Source: CAD feature listing. Evaluate the final solid. Frame: model axes, mm. A direction names the side the tool comes from. Round coordinates to 2 decimals unless told otherwise and drop trailing zeros. Loops run counter-clockwise (first coordinate to the right, second up) from the corner with the lowest first, then second, coordinate; pieces in that order, holes last. Notation, with made-up numbers: (-28, 53.25) - (-10, 53.25) arc R10 ccw to (-10, 72.25) - close; hole circle Ø7 at (-39.75, 32.5). An arc over 180 degrees is marked (long way). One line per question, with ' | ' between items.
from build123d import *

# Parameters (mm, degrees)
F0_R     = 2.65
F0_R_2   = 3.5
F1_DEPTH = 9.5
F2_DEPTH = 6.35
F3_DEPTH = 9.501


with BuildPart() as f1:
    # F0 (on Top) → F1 (new body)
    with BuildSketch(Plane.XY):
        with Locations((4.775, -2.49704)):
            Circle(F0_R)
        with Locations((5, -2.886751)):
            Circle(F0_R_2)
        with Locations((4.775, -2.49704)):
            Circle(F0_R, mode=Mode.SUBTRACT)
    extrude(amount=F1_DEPTH)

    # F0 (on Top) → F2 (join)
    with BuildSketch(Plane.XY):
        Polygon((1.633975, 0.943376), (0, 0), (0, -5.773503), (5, -8.660254), (10, -5.773503), (10, 0), (5, 2.886751), (3.366025, 1.943376), (3, 0.57735), align=None)
        with Locations((5, -2.886751)):
            Circle(F0_R_2, mode=Mode.SUBTRACT)
    extrude(amount=F2_DEPTH)

    # F0 (on Top) → F3 (cut, through all)
    with BuildSketch(Plane.XY):
        with Locations((4.775, -2.49704)):
            Circle(F0_R)
    extrude(amount=F3_DEPTH, mode=Mode.SUBTRACT)


solid = f1.part
1. Section query A-A, the plane x = 2.75. Return loops of the section in (y, z).
Worked out:
outline: (-7.36, 0) - (-4.21, 0) - (-4.21, 9.5) - (-5.57, 9.5) - (-5.57, 6.35) - (-7.36, 6.35) - close; (-0.79, 0) - (0.64, 0) - (0.64, 6.35) - (-0.21, 6.35) - (-0.21, 9.5) - (-0.79, 9.5) - close
2. Contact query for flat-ended pins moving along their axis: P1, Ø1, axis at x = 3, z = 2.5, coming from the -Y side; P2, Ø5, axis at x = 4.78, y = -2.5, coming from the +Z side; P3, Ø1.5, axis at y = -2.5, z = 8.5, coming from the +X side. Output: stop coordinate, or through.
Worked out:
P1: stops at y = -7.79 | P2: passes through | P3: stops at x = 8.5
3. Material intervals for probe 1 along Z at (x, y) = (7, -6.75); probe 2 along X at (y, z) = (-3, 4.5); probe 3 along X at (y, z) = (-3.75, 2.25), sorted ascending.
Worked out:
probe 1: z = 0 to 6.35 | probe 2: x = 0 to 2.17, 7.38 to 10 | probe 3: x = 0 to 2.44, 7.11 to 10
4. Section query D-D, the plane x = 8. Return loops of the section in (y, z), plus the area to 3 significant figures.
Worked out:
outline: (-6.93, 0) - (1.15, 0) - (1.15, 6.35) - (-1.08, 6.35) - (-1.08, 9.5) - (-4.69, 9.5) - (-4.69, 6.35) - (-6.93, 6.35) - close | area: 62.7 mm2
5. Mould query, pull axis X, two halves, no side actions, for faces 3 (the cylindrical face through (8.23, -4.23, 7.9)), 4 (the flat face through (5, -7, 6.35)), 5 (the cylindrical face through (7.303, -1.701, 4.684)), 6 (the flat face through (2.327, 0.758, 3.131)). Classes: released by +X, released by -X, zero draft, split by the parting line, or undercut.
Worked out:
face 3: split by the parting line | face 4: zero draft | face 5: undercut | face 6: undercut
6. Section query B-B, the plane y = -4. Return loops of the section in (x, z).
Worked out:
outline: (0, 0) - (2.59, 0) - (2.59, 9.5) - (1.68, 9.5) - (1.68, 6.35) - (0, 6.35) - close; (6.96, 0) - (10, 0) - (10, 6.35) - (8.32, 6.35) - (8.32, 9.5) - (6.96, 9.5) - close
7. Access query for faces 1 (the flat face through (3.186, 1.27, 3.131)), 2 (the flat face through (5.502, -5.204, 9.5)). Directions: +Z, -Z, +X, -X, +Y, -Y. A direction counts if a zero-diameter tool reaches every point of the face in a straight line with its end or side. Return the directions, or none.
Worked out:
face 1: +Z, -Z, +Y | face 2: +Z, +X, -X, +Y, -Y
